For this review, use the dimensioned drawing (mm, ordinates from the lowest corner) and the shaded views. A direction names the side the tool comes from. Round coordinates to 2 decimals unless told otherwise and drop trailing zeros. Write each loop counter-clockwise with the first axis right and the second up, starting at its lowest first coordinate (ties: lowest second). Pieces come first, ordered by that corner, then holes. Notation, with made-up numbers: M -10.75,70.25 L 3.25,70.25 A14 ccw 3.25,91.25 Z; hole C -28.5,-1.5 d5. An arc over 180 degrees is marked long. One line per question, with ' | ' between items. Start each with the question number.
Item 1: Add section C-C, the plane x = 19.05. State the section outline as (y, z) points (3 decimals), and give its area (3 significant figures).
Item 2: Insertion check: pin 1 Ø12 at (x, z) = (23, 14.5) entering from -Y (3 decimals). The pin has a flat end and moves straight along its axis. Give the tip position at first contact, or say it passes through.
Item 3: Draft analysis for pull direction Z (two halves, no side actions). For the marked faces 3, 4, 5 and 6, state which applies: released by +Z, released by -Z, zero draft, split by the parting line, or undercut.
Item 4: Add section D-D, the plane x = 9.5. State the section outline as (y, z) points (3 decimals), and give its area (3 significant figures).
Item 5: Machinability: for the marked faces 1 and 2, which of the approach directions +Z, -Z, +X, -X, +Y, -Y give a long, thin tool a straight path to every point of the face, cutting with its end or side? Answer none if there is none.
Item 6: For L1, parallel to Z at x = 18.5, y = 1; L2, parallel to Y at x = 10, z = 6 (3 decimals); L3, parallel to Z at x = 14.5, y = 9, list the stretches that pass through material, from the lowest coordinate up.
Item 7: Add section A-A, the plane y = 6.25. State the section outline as (x, z) points, and give its area (3 significant figures).
Item 8: Add section B-B, the plane z = 12.7. State the section outline as (x, y) points (3 decimals), and give its area (3 significant figures).
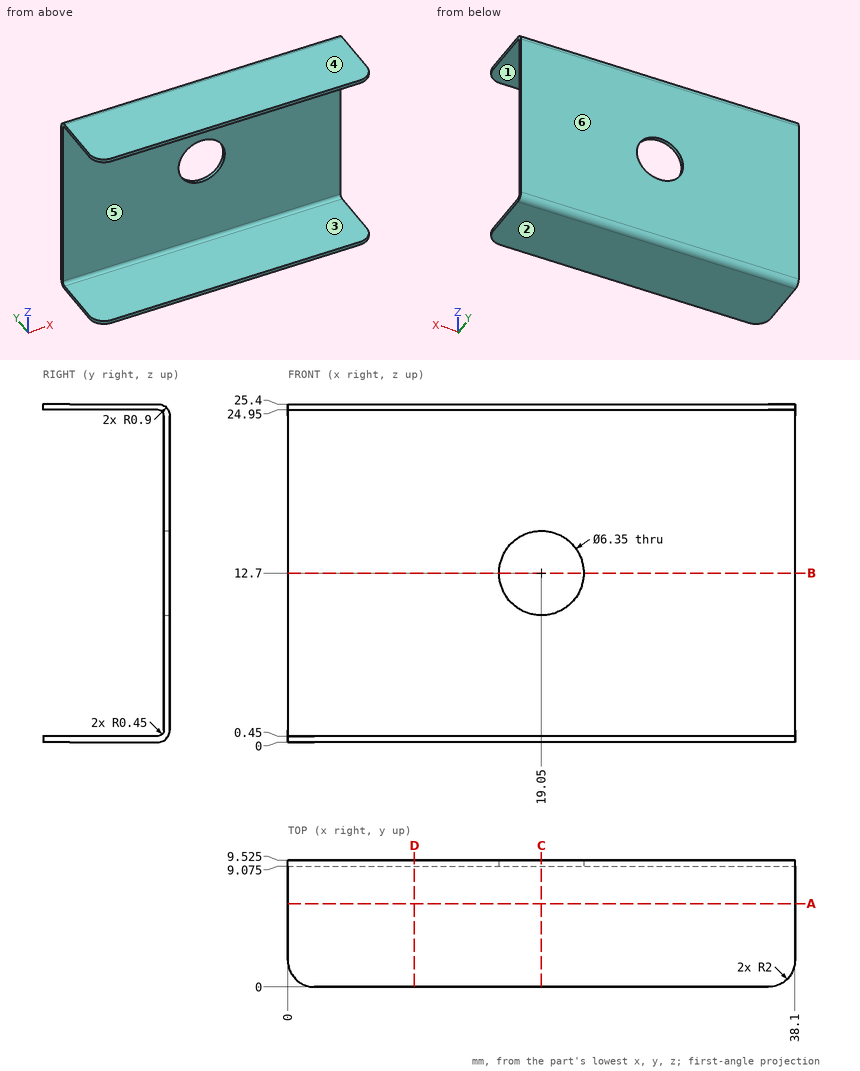
Computed values:
1) outline: M 0,0 L 8.625,0 A0.9 ccw 9.525,0.9 L 9.525,9.525 L 9.075,9.525 L 9.075,0.9 A0.45 cw 8.625,0.45 L 0,0.45 Z; M 0,24.95 L 8.625,24.95 A0.45 cw 9.075,24.5 L 9.075,15.875 L 9.525,15.875 L 9.525,24.5 A0.9 ccw 8.625,25.4 L 0,25.4 Z | area: 16.5 mm^2
2) pin 1: stops at y = 9.075
3) face 3: undercut | face 4: released by +Z | face 5: undercut | face 6: zero draft
4) outline: M 0,0 L 8.625,0 A0.9 ccw 9.525,0.9 L 9.525,24.5 A0.9 ccw 8.625,25.4 L 0,25.4 L 0,24.95 L 8.625,24.95 A0.45 cw 9.075,24.5 L 9.075,0.9 A0.45 cw 8.625,0.45 L 0,0.45 Z | area: 19.3 mm^2
5) face 1: +X, -X, -Y | face 2: -Z, +X, -X, +Y, -Y
6) L1: z = 0 to 0.45, 24.95 to 25.4 | L2: y = 9.075 to 9.525 | L3: z = 0.08 to 0.65, 24.75 to 25.32
7) outline: M 0,0 L 38.1,0 L 38.1,0.45 L 0,0.45 Z; M 0,24.95 L 38.1,24.95 L 38.1,25.4 L 0,25.4 Z | area: 34.3 mm^2
8) outline: M 0,9.075 L 15.875,9.075 L 15.875,9.525 L 0,9.525 Z; M 22.225,9.075 L 38.1,9.075 L 38.1,9.525 L 22.225,9.525 Z | area: 14.3 mm^2
